```python
from build123d import *

# Parameters (mm, degrees)
BOSS_EXTRUDE1_DEPTH = 6.125
BOSS_EXTRUDE2_DEPTH = 3.8
BOSS_EXTRUDE3_DEPTH = 0.7
SKETCH4_R           = 1
CUT_EXTRUDE1_DEPTH  = 11.5
SKETCH5_R           = 0.975
CUT_EXTRUDE2_DEPTH  = 1
SKETCH6_R           = 0.5
BOSS_EXTRUDE4_DEPTH = 8
SKETCH7_R           = 0.25
BOSS_EXTRUDE5_DEPTH = 1
BOSS_EXTRUDE6_DEPTH = 0.6
SKETCH9_W           = 1.425
SKETCH9_H           = 3.2
FILLET1_R           = 0.3
FILLET2_R           = 2
FILLET3_R           = 0.5


with BuildPart() as part:
    # Sketch1 → Boss-Extrude1 (new body, symmetric)
    with BuildSketch(Plane.XY):
        Polygon((-7.13, 6), (11.92, 6), (16.62, 5.1), (16.62, 1.85), (20.87, 1.85), (20.87, 0), (16.62, 0), (16.62, -15.6), (-7.13, -15.6), (-7.13, 0), (-11.38, 0), (-11.38, 1.85), (-7.13, 1.85), align=None)
    extrude(amount=BOSS_EXTRUDE1_DEPTH, both=True)

    # Sketch2 → Boss-Extrude2 (add)
    with BuildSketch(Plane(origin=(0, 6, 0), x_dir=(1, 0, 0), z_dir=(0, 1, 0))):
        with BuildLine():
            Line((5.251487884, -2.85), (6.125, -2.85))
            ThreePointArc((6.125, -2.85), (8.975, 0), (6.125, 2.85))
            Line((6.125, 2.85), (5.251487884, 2.85))
            ThreePointArc((5.251487884, 2.85), (-5.975, 0), (5.251487884, -2.85))
        make_face()
    extrude(amount=BOSS_EXTRUDE2_DEPTH)

    # Sketch3 → Boss-Extrude3 (add)
    with BuildSketch(Plane(origin=(0, 9.8, 0), x_dir=(1, 0, 0), z_dir=(0, 1, 0))):
        with BuildLine():
            Line((4.498263554, -1.675), (6.125, -1.675))
            ThreePointArc((6.125, -1.675), (7.8, 0), (6.125, 1.675))
            Line((6.125, 1.675), (4.498263554, 1.675))
            ThreePointArc((4.498263554, 1.675), (-4.8, 0), (4.498263554, -1.675))
        make_face()
    extrude(amount=BOSS_EXTRUDE3_DEPTH)

    # Sketch4 → Cut-Extrude1 (cut, through all)
    with BuildSketch(Plane(origin=(0, 0, 0), x_dir=(1, 0, 0), z_dir=(0, 1, 0))):
        with Locations((-9.505, 3.5)):
            Circle(SKETCH4_R)
        with Locations((-9.505, -3.5)):
            Circle(SKETCH4_R)
        with Locations((18.995, 3.5)):
            Circle(SKETCH4_R)
        with Locations((18.995, -3.5)):
            Circle(SKETCH4_R)
        with Locations((18.995, 0)):
            Circle(SKETCH4_R)
        with Locations((-9.505, 0)):
            Circle(SKETCH4_R)
    extrude(amount=CUT_EXTRUDE1_DEPTH, mode=Mode.SUBTRACT)

    # Sketch5 → Cut-Extrude2 (cut)
    with BuildSketch(Plane.XZ.offset(15.6)):
        with BuildLine():
            Line((16.62, 6.125), (13.995, 6.125))
            Line((13.995, 6.125), (13.995, 4.85))
            ThreePointArc((13.995, 4.85), (14.375761184, 3.930761184), (15.295, 3.55))
            Line((15.295, 3.55), (16.62, 3.55))
            Line((16.62, 3.55), (16.62, 6.125))
        make_face()
        with Locations((15.395, 4.95)):
            Circle(SKETCH5_R, mode=Mode.SUBTRACT)
        with BuildLine():
            Line((16.62, -6.125), (13.995, -6.125))
            Line((13.995, -6.125), (13.995, -4.85))
            ThreePointArc((13.995, -4.85), (14.375761184, -3.930761184), (15.295, -3.55))
            Line((15.295, -3.55), (16.62, -3.55))
            Line((16.62, -3.55), (16.62, -6.125))
        make_face()
        with Locations((15.395, -4.95)):
            Circle(SKETCH5_R, mode=Mode.SUBTRACT)
        with BuildLine():
            Line((-7.13, 6.125), (-4.505, 6.125))
            Line((-4.505, 6.125), (-4.505, 4.85))
            ThreePointArc((-4.505, 4.85), (-4.885761184, 3.930761184), (-5.805, 3.55))
            Line((-5.805, 3.55), (-7.13, 3.55))
            Line((-7.13, 3.55), (-7.13, 6.125))
        make_face()
        with Locations((-5.905, 4.95)):
            Circle(SKETCH5_R, mode=Mode.SUBTRACT)
        with BuildLine():
            Line((-7.13, -6.125), (-4.505, -6.125))
            Line((-4.505, -6.125), (-4.505, -4.85))
            ThreePointArc((-4.505, -4.85), (-4.885761184, -3.930761184), (-5.805, -3.55))
            Line((-5.805, -3.55), (-7.13, -3.55))
            Line((-7.13, -3.55), (-7.13, -6.125))
        make_face()
        with Locations((-5.905, -4.95)):
            Circle(SKETCH5_R, mode=Mode.SUBTRACT)
    extrude(amount=-CUT_EXTRUDE2_DEPTH, mode=Mode.SUBTRACT)

    # Sketch6 → Boss-Extrude4 (add)
    with BuildSketch(Plane.ZY.offset(7.13)):
        with Locations((0, -11.7)):
            Circle(SKETCH6_R)
        with Locations((1.05, -11.7)):
            Circle(SKETCH6_R)
        with Locations((-1.05, -11.7)):
            Circle(SKETCH6_R)
    extrude(amount=BOSS_EXTRUDE4_DEPTH)

    # Sketch7 → Boss-Extrude5 (add)
    with BuildSketch(Plane.ZY.offset(15.13)):
        with Locations((0, -11.7)):
            Circle(SKETCH7_R)
        with Locations((1.05, -11.7)):
            Circle(SKETCH7_R)
        with Locations((-1.05, -11.7)):
            Circle(SKETCH7_R)
    extrude(amount=BOSS_EXTRUDE5_DEPTH)

    # Sketch8 → Boss-Extrude6 (add, symmetric)
    with BuildSketch(Plane.XY):
        Polygon((11.92, 6), (7.8, 6.78893617), (7.8, 6), align=None)
    extrude(amount=BOSS_EXTRUDE6_DEPTH, both=True)

    # Sketch9 → Revolve1 (revolve)
    with BuildSketch(Plane.XY):
        with Locations((1.7125, 12.1)):
            Rectangle(SKETCH9_W, SKETCH9_H)
    revolve(axis=Axis((0, 55, 0), (0, -1, 0)))

    # Fillet1
    fillet1_edges = [part.edges().sort_by_distance(p)[0] for p in [
        (14.42, -15.6, -4.95),
        (-6.88, -15.6, 4.95),
        (-6.88, -15.6, -4.95),
        (14.42, -15.6, 4.95),
    ]]
    fillet(fillet1_edges, radius=FILLET1_R)

    # Fillet2
    fillet2_edges = [part.edges().sort_by_distance(p)[0] for p in [
        (-11.38, 0.925, 6.125),
        (20.87, 0.925, -6.125),
        (-11.38, 0.925, -6.125),
        (20.87, 0.925, 6.125),
    ]]
    fillet(fillet2_edges, radius=FILLET2_R)

    # Fillet3
    fillet3_edges = [part.edges().sort_by_distance(p)[0] for p in [
        (16.62, -7.3, -6.125),
        (16.62, 3.475, -6.125),
        (-7.13, -7.3, -6.125),
        (-7.13, -7.3, 6.125),
        (-7.13, 3.925, -6.125),
        (16.62, 3.475, 6.125),
        (-7.13, 3.925, 6.125),
        (16.62, -7.3, 6.125),
    ]]
    fillet(fillet3_edges, radius=FILLET3_R)


solid = part.part
```
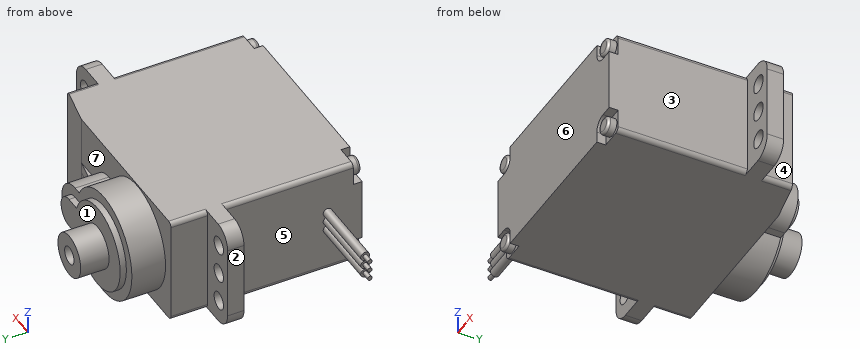
Work out the finished part from the listing and answer in its coordinate system (mm). Face numbers are marked on the shaded views. A direction names the side the tool comes from. Coordinates: 2 decimals unless noted, no trailing zeros. Loops run counter-clockwise (first coordinate to the right, second up) from the corner with the lowest first, then second, coordinate; pieces in that order, holes last. Notation, with made-up numbers: M 0,82 L 17,82 A33 ccw 17,110 Z; hole C 61,36 d5. An arc over 180 degrees is marked long. Use CSV: the item, a comma, the result in double quotes. Start each with the question number.
(1) For the marked faces 1, 2, 3 and 4, determine the directions among +Z, -Z, +X, -X, +Y, -Y from which every point of the face is accessible in a straight line to the end or side of a thin tool.
(2) Given pin 1 Ø1 at (y, z) = (-2.5, 1) entering from -X; pin 2 Ø1 at (x, z) = (0, 0) entering from +Y; pin 3 Ø1.4 at (x, z) = (-9, 2.5) entering from +Y, each flat-ended and moving along its own axis, determine where each tip first touches the part or whether it passes through.
(3) Find section B-B, the plane x = 0. Give the vertices of the cut face in (y, z) (3 decimals), then the cut area to 3 significant figures.
(4) For a pull along Y with two mould halves and no side action, classify the marked faces 5, 6 and 7 as +Y half, -Y half, draft (parallel to the pull), parting line (faces both ways), or undercut.
(5) Consider line 1 (X direction, y = 0.7, z = 0) (3 decimals); line 2 (Z direction, x = 0, y = 12.05) (3 decimals); line 3 (X direction, y = -8.25, z = -1.5). Determine where each line is inside the solid, lowest interval first.
(6) Find section A-A, the plane y = 4.25. Give the vertices of the cut face in (x, z) (3 decimals), then the cut area to 3 significant figures.
Recorded:
1,face 1,"+Y"
1,face 2,"+Z, -Z, -X, +Y"
1,face 3,"+Z, -Z, +X, -Y"
1,face 4,"+Z, -Z, +X, +Y"
2,pin 1,"stops at x = -7.13"
2,pin 2,"stops at y = 10.5"
2,pin 3,"stops at y = 1.85"
3,outline,"M -15.6,-6.125 L 6,-6.125 L 6,-5.975 L 9.8,-5.975 L 9.8,-4.8 L 10.5,-4.8 L 10.5,-2.425 L 13.7,-2.425 L 13.7,-1 L 10.5,-1 L 10.5,1 L 13.7,1 L 13.7,2.425 L 10.5,2.425 L 10.5,4.8 L 9.8,4.8 L 9.8,5.975 L 6,5.975 L 6,6.125 L -15.6,6.125 Z"
3,area,"326 mm^2"
4,face 5,"undercut"
4,face 6,"-Y half"
4,face 7,"+Y half"
5,line 1,"x = -11.38 to -10.505, -8.505 to 17.995, 19.995 to 20.87"
5,line 2,"z = -2.425 to -1, 1 to 2.425"
5,line 3,"x = -7.13 to 16.62"
6,outline,"M -7.13,-5.625 A0.5 ccw -6.63,-6.125 L 16.12,-6.125 A0.5 ccw 16.62,-5.625 L 16.62,5.625 A0.5 ccw 16.12,6.125 L -6.63,6.125 A0.5 ccw -7.13,5.625 Z"
6,area,"291 mm^2"
